Part model, mm, in its own coordinate system. A direction names the side the tool comes from. Give positions to 0.01 mm unless a question says otherwise; leave off trailing zeros. Order: outer loops, then holes, each group sorted by start corner. A loop starts at its lowest first (then second) coordinate and runs counter-clockwise, first axis right, second up. Notation, with made-up numbers: (24, -31.5) - (37, -31.5) arc R6 ccw to (37, -27.5) - close; hole circle Ø2 at (28, 75.25). An arc over 180 degrees is marked (long way). One line per item, written item: value.
```python
from build123d import *

# Parameters (mm, degrees)
SKETCH1_W           = 45
SKETCH1_H           = 31
SKETCH1_R           = 5.25
SKETCH1_R_2         = 2
BOSS_EXTRUDE1_DEPTH = 20
SKETCH2_R           = 2
CUT_EXTRUDE1_DEPTH  = 32
SKETCH3_W           = 9.5
SKETCH3_H           = 16
CUT_EXTRUDE2_DEPTH  = 21


with BuildPart() as part:
    # Sketch1 → Boss-Extrude1 (new body)
    with BuildSketch(Plane.XY):
        with Locations((0, -0.5)):
            Rectangle(SKETCH1_W, SKETCH1_H)
        Circle(SKETCH1_R, mode=Mode.SUBTRACT)
        with Locations((0, 8)):
            Circle(SKETCH1_R_2, mode=Mode.SUBTRACT)
        with Locations((8, 0)):
            Circle(SKETCH1_R_2, mode=Mode.SUBTRACT)
        with Locations((0, -8)):
            Circle(SKETCH1_R_2, mode=Mode.SUBTRACT)
        with Locations((-8, 0)):
            Circle(SKETCH1_R_2, mode=Mode.SUBTRACT)
    extrude(amount=BOSS_EXTRUDE1_DEPTH)

    # Sketch2 → Cut-Extrude1 (cut, through all)
    with BuildSketch(Plane(origin=(0, 15, 0), x_dir=(1, 0, 0), z_dir=(0, 1, 0))):
        with Locations((-17.5, -10)):
            Circle(SKETCH2_R)
        with Locations((17.5, -10)):
            Circle(SKETCH2_R)
    extrude(amount=-CUT_EXTRUDE1_DEPTH, mode=Mode.SUBTRACT)

    # Sketch3 → Cut-Extrude2 (cut, through all)
    with BuildSketch(Plane(origin=(0, 0, 0), x_dir=(-1, 0, 0), z_dir=(0, 0, -1))):
        with Locations((17.75, 7)):
            Rectangle(SKETCH3_W, SKETCH3_H)
        with Locations((-17.75, 7)):
            Rectangle(SKETCH3_W, SKETCH3_H)
    extrude(amount=-CUT_EXTRUDE2_DEPTH, mode=Mode.SUBTRACT)


solid = part.part
```
1) Slice it at C-C on y = 0. Write the cut outline in (x, z), then the cut area to 3 significant figures.
Answer:
outline: (-13, 0) - (-10, 0) - (-10, 20) - (-13, 20) - close; (-6, 0) - (-5.25, 0) - (-5.25, 20) - (-6, 20) - close; (5.25, 0) - (6, 0) - (6, 20) - (5.25, 20) - close; (10, 0) - (13, 0) - (13, 20) - (10, 20) - close
area: 150 mm2
2) Slice it at D-D on x = 0. Write the cut outline in (y, z), then the cut area to 3 significant figures.
Answer:
outline: (-16, 0) - (-10, 0) - (-10, 20) - (-16, 20) - close; (-6, 0) - (-5.25, 0) - (-5.25, 20) - (-6, 20) - close; (5.25, 0) - (6, 0) - (6, 20) - (5.25, 20) - close; (10, 0) - (15, 0) - (15, 20) - (10, 20) - close
area: 250 mm2
3) Wall check: line 1 along Y through (x, z) = (0, 9.75); line 2 along Z through (x, y) = (17.5, -5); line 3 along Y through (x, z) = (8, 15.25). Give the ranges that are in metal, low to high. Write a range as [from, to].
Answer:
line 1: y = [-16, -10], [-6, -5.25], [5.25, 6], [10, 15]
line 2: z = [0, 8], [12, 20]
line 3: y = [-16, -2], [2, 15]
4) Slice it at A-A on y = -8. Write the cut outline in (x, z), then the cut area to 3 significant figures.
Answer:
outline: (-22.5, 0) - (-2, 0) - (-2, 20) - (-22.5, 20) - close; (2, 0) - (22.5, 0) - (22.5, 20) - (2, 20) - close; hole circle Ø4 at (-17.5, 10); hole circle Ø4 at (17.5, 10)
area: 795 mm2
5) Drop flat-ended pins along their axis: P1, Ø2.5, axis at x = 0, y = -8, coming from the -Z side; P2, Ø1.5, axis at y = 4, z = 15.5, coming from the +X side; P3, Ø3, axis at x = 17, z = 8.5, coming from the +Y side. Give the stop position or say it passes through.
Answer:
P1: passes through
P2: stops at x = 13
P3: stops at y = -1
6) Two-plate mould, pull along X, no slides. Class faces 1 (the face through (0, -6, 10)), 2 (the face through (-20, -1, 10)), 3 (the face through (16.026, -8.395, 8.648)), 4 (the face through (13, 7, 10)): pulls with the +X half, pulls with the -X half, needs draft (parallel to the pull), parting line crosses it, or undercut.
Answer:
face 1: undercut
face 2: needs draft
face 3: undercut
face 4: pulls with the +X half
7) Which spindle directions (+Z, -Z, +X, -X, +Y, -Y) get a long thin tool onto all of the face, cutting with end or side? Do faces 5 (the face through (-18.974, -8.395, 8.648)), 6 (the face through (20, -1, 10)), 7 (the face through (-13, 7, 10)). Say none if no direction does.
Answer:
face 5: +Y, -Y
face 6: +Z, -Z, +X, +Y
face 7: +Z, -Z, -X, +Y
8) Slice it at B-B on x = 8. Write the cut outline in (y, z).
Answer:
outline: (-16, 0) - (-2, 0) - (-2, 20) - (-16, 20) - close; (2, 0) - (15, 0) - (15, 20) - (2, 20) - close
